For this review, take the finished solid that the model builds, in its own axes (mm). Round coordinates to 2 decimals unless told otherwise and drop trailing zeros. Loops run counter-clockwise (first coordinate to the right, second up) from the corner with the lowest first, then second, coordinate; pieces in that order, holes last. Notation, with made-up numbers: (-25.5, -26) -> (23.5, -26) arc R22 ccw to (23.5, 9) -> close; hole circle Ø11 at (-7, 52.25). An arc over 180 degrees is marked (long way). One line per question, with ' | ' between items. Start each with the question number.
1. Wall thickness on line 1 along X through (y, z) = (-4, 6); line 2 along Y through (x, z) = (-0.25, 6.5); line 3 along Z through (x, y) = (5, -3.25): over which ranges is each line inside the solid? List them lowest first.
2. Consider section C-C (z = 1). Write out the cut boundary in (x, y), and give its area (3 significant figures).
3. Draft analysis for pull direction X (two halves, no side actions). For faces 1 (the face through (5.334, -3, 5.8)), 2 (the face through (0, 0.508, 0)), 3 (the face through (0.254, -3.1, 5.8)), 4 (the face through (-5.334, -3, 5.8)), state which applies: pulls with the +X half, pulls with the -X half, needs draft (parallel to the pull), parting line crosses it, or undercut.
4. For pin 1 Ø1.5 at (x, z) = (1.5, 4.5) entering from -Y; pin 2 Ø1 at (y, z) = (-4, 5.5) entering from +X; pin 3 Ø0.6 at (x, y) = (5, -1.5) entering from +Z, all flat-tipped, find the tip position at first contact; note any pin that passes through.
5. Consider section A-A (z = 5.08). Write out the cut boundary in (x, y).
6. Consider section B-B (x = 6.25). Write out the cut boundary in (y, z), and give its area (3 significant figures).
Autodesk Inventor part; units mm, degrees
ref_plane "pole_to_body_XY" through (0, 0.508, 0) normal (0, 1, 0) x (1, 0, 0)
ref_plane "pole_to_body_YZ" through (0, 0.508, 0) normal (1, 0, 0) x (0, 0, -1)
ref_plane "pole_to_body_ZX" through (0, 0.508, 0) normal (0, 0, -1) x (0, 1, 0)
sketch "Sketch_1" plane through (0, 0, 0) normal (0, 1, 0) x (-1, 0, 0)
  line L0 (7.112, -7.112) -> (7.112, 7.112)
  line L1 (7.112, 7.112) -> (-7.112, 7.112)
  line L2 (-7.112, 7.112) -> (-7.112, -7.112)
  line L3 (-7.112, -7.112) -> (7.112, -7.112)
extrude "Extrusion1" add sketch "Sketch_1" along normal blind 0.508
sketch "Sketch_2" plane through (-5.08, 0, 0) normal (1, 0, 0) x (0, 0, -1)
  line L0 (-6.0833, -4.9859) -> (-5.4864, -6.0198)
  line L1 (-5.4864, -6.0198) -> (-4.6736, -6.0198)
  line L2 (-4.6736, -6.0198) -> (-4.0767, -4.9859)
  line L3 (-4.0767, -4.9859) -> (-4.0767, 0.508)
  line L4 (-4.0767, 0.508) -> (-6.0833, 0.508)
  line L5 (-6.0833, 0.508) -> (-6.0833, -4.9859)
  line L6 (-5.4864, -2.3622) -> (-5.4864, -3.1496)
  arc A0 (-5.4864, -3.1496) -> (-5.08, -3.556) centre (-5.08, -3.1496) ccw
  arc A1 (-5.08, -3.556) -> (-4.6736, -3.1496) centre (-5.08, -3.1496) ccw
  line L7 (-4.6736, -3.1496) -> (-4.6736, -2.3622)
  arc A2 (-4.6736, -2.3622) -> (-5.08, -1.9558) centre (-5.08, -2.3622) ccw
  arc A3 (-5.08, -1.9558) -> (-5.4864, -2.3622) centre (-5.08, -2.3622) ccw
extrude "Extrusion2" add sketch "Sketch_2" along normal mid plane 0.508
sketch "Sketch_4" plane through (0, 0, 0) normal (1, 0, 0) x (0, 1, 0)
  line L0 (-4.9859, 6.0833) -> (-6.0198, 5.4864)
  line L1 (-6.0198, 5.4864) -> (-6.0198, 4.6736)
  line L2 (-6.0198, 4.6736) -> (-4.9859, 4.0767)
  line L3 (-4.9859, 4.0767) -> (0.508, 4.0767)
  line L4 (0.508, 4.0767) -> (0.508, 6.0833)
  line L5 (0.508, 6.0833) -> (-4.9859, 6.0833)
  line L6 (-2.3622, 5.4864) -> (-3.1496, 5.4864)
  arc A0 (-3.1496, 5.4864) -> (-3.556, 5.08) centre (-3.1496, 5.08) ccw
  arc A1 (-3.556, 5.08) -> (-3.1496, 4.6736) centre (-3.1496, 5.08) ccw
  line L7 (-3.1496, 4.6736) -> (-2.3622, 4.6736)
  arc A2 (-2.3622, 4.6736) -> (-1.9558, 5.08) centre (-2.3622, 5.08) ccw
  arc A3 (-1.9558, 5.08) -> (-2.3622, 5.4864) centre (-2.3622, 5.08) ccw
extrude "Extrusion3" add sketch "Sketch_4" along normal mid plane 0.508
sketch "Sketch_6" plane through (5.08, 0, 0) normal (1, 0, 0) x (0, 0, -1)
  line L0 (-6.0833, -4.9859) -> (-5.4864, -6.0198)
  line L1 (-5.4864, -6.0198) -> (-4.6736, -6.0198)
  line L2 (-4.6736, -6.0198) -> (-4.0767, -4.9859)
  line L3 (-4.0767, -4.9859) -> (-4.0767, 0.508)
  line L4 (-4.0767, 0.508) -> (-6.0833, 0.508)
  line L5 (-6.0833, 0.508) -> (-6.0833, -4.9859)
  line L6 (-5.4864, -2.3622) -> (-5.4864, -3.1496)
  arc A0 (-5.4864, -3.1496) -> (-5.08, -3.556) centre (-5.08, -3.1496) ccw
  arc A1 (-5.08, -3.556) -> (-4.6736, -3.1496) centre (-5.08, -3.1496) ccw
  line L7 (-4.6736, -3.1496) -> (-4.6736, -2.3622)
  arc A2 (-4.6736, -2.3622) -> (-5.08, -1.9558) centre (-5.08, -2.3622) ccw
  arc A3 (-5.08, -1.9558) -> (-5.4864, -2.3622) centre (-5.08, -2.3622) ccw
extrude "Extrusion4" add sketch "Sketch_6" along normal mid plane 0.508
ref_plane "pole_to_body_XY" through (0, 0.508, 0) normal (0, 1, 0) x (1, 0, 0)
ref_plane "pole_to_body_YZ" through (0, 0.508, 0) normal (1, 0, 0) x (0, 0, -1)
ref_plane "pole_to_body_ZX" through (0, 0.508, 0) normal (0, 0, -1) x (0, 1, 0)
properties part number "UB216KKW015C-NR"
Answer block:
1) line 1: x = -5.33 to -4.83, -0.25 to 0.25, 4.83 to 5.33 | line 2: y = 0 to 0.51 | line 3: z = 4.08 to 4.69, 5.47 to 6.08
2) outline: (-7.11, 0) -> (7.11, 0) -> (7.11, 0.51) -> (-7.11, 0.51) -> close | area: 7.23 mm2
3) face 1: pulls with the +X half | face 2: needs draft | face 3: undercut | face 4: pulls with the -X half
4) pin 1: stops at y = 0 | pin 2: stops at x = 5.33 | pin 3: stops at z = 6.08
5) outline: (-7.11, 0) -> (-5.33, 0) -> (-5.33, -1.96) -> (-4.83, -1.96) -> (-4.83, 0) -> (-0.25, 0) -> (-0.25, -1.96) -> (0.25, -1.96) -> (0.25, 0) -> (4.83, 0) -> (4.83, -1.96) -> (5.33, -1.96) -> (5.33, 0) -> (7.11, 0) -> (7.11, 0.51) -> (-7.11, 0.51) -> close; (-5.33, -6.02) -> (-4.83, -6.02) -> (-4.83, -3.56) -> (-5.33, -3.56) -> close; (-0.25, -6.02) -> (0.25, -6.02) -> (0.25, -3.56) -> (-0.25, -3.56) -> close; (4.83, -6.02) -> (5.33, -6.02) -> (5.33, -3.56) -> (4.83, -3.56) -> close
6) outline: (0, -7.11) -> (0.51, -7.11) -> (0.51, 7.11) -> (0, 7.11) -> close | area: 7.23 mm2
